Build history of the part. All positions in model axes, mm. Face numbers are marked on the shaded views. Give positions to 0.01 mm unless a question says otherwise; leave off trailing zeros. Order: outer loops, then holes, each group sorted by start corner. A loop starts at its lowest first (then second) coordinate and runs counter-clockwise, first axis right, second up. Notation, with made-up numbers: (44.5, -18.75) - (56.5, -18.75) arc R18 ccw to (56.5, -10.75) - close; hole circle Ø2 at (4.25, 23). An arc over 180 degrees is marked (long way). Answer in a Markdown table with one row per item.
```python
from build123d import *

# Parameters (mm, degrees)
F0_W     = 88.9
F0_H     = 88.9
F0_R     = 1.9812
F0_R_2   = 29.845
F1_DEPTH = 19.05
F2_R     = 3.175
F3_DEPTH = 25.4
F4_R     = 3.175
F5_DEPTH = 25.4


with BuildPart() as f1:
    # F0 (on Top) → F1 (new body)
    with BuildSketch(Plane.XY):
        Rectangle(F0_W, F0_H)
        with Locations((-38.1, -38.1)):
            Circle(F0_R, mode=Mode.SUBTRACT)
        with Locations((38.1, -38.1)):
            Circle(F0_R, mode=Mode.SUBTRACT)
        with Locations((-38.1, 38.1)):
            Circle(F0_R, mode=Mode.SUBTRACT)
        Circle(F0_R_2, mode=Mode.SUBTRACT)
        with Locations((38.1, 38.1)):
            Circle(F0_R, mode=Mode.SUBTRACT)
    extrude(amount=F1_DEPTH)

    # F2 (on face) → F3 (cut)
    with BuildSketch(Plane(origin=(0, 44.45, 0), x_dir=(-1, 0, 0), z_dir=(0, 1, 0))):
        with Locations((0, 9.525)):
            Circle(F2_R)
    extrude(amount=-F3_DEPTH, mode=Mode.SUBTRACT)

    # F4 (on face) → F5 (cut)
    with BuildSketch(Plane(origin=(-44.45, 0, 0), x_dir=(0, -1, 0), z_dir=(-1, 0, 0))):
        with Locations((0, 9.525)):
            Circle(F4_R)
    extrude(amount=-F5_DEPTH, mode=Mode.SUBTRACT)


solid = f1.part
```
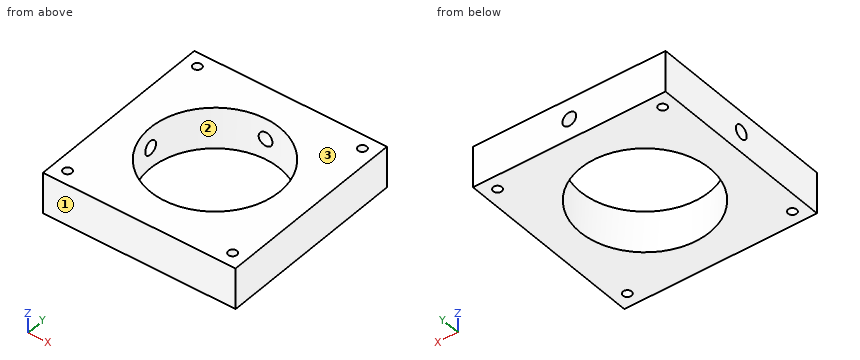
1. Cut at D-D on x = 0. Write the cut outline in (y, z) (3 decimals).
Check result:
| item | result |
|---|---|
| outline | (-44.45, 0) - (-29.845, 0) - (-29.845, 19.05) - (-44.45, 19.05) - close; (29.845, 0) - (44.45, 0) - (44.45, 6.35) - (29.845, 6.35) - close; (29.845, 12.7) - (44.45, 12.7) - (44.45, 19.05) - (29.845, 19.05) - close |
2. Cut at C-C on y = 38.1. Write the cut outline in (x, z) (3 decimals).
Check result:
| item | result |
|---|---|
| outline | (-44.45, 0) - (-40.081, 0) - (-40.081, 19.05) - (-44.45, 19.05) - close; (-36.119, 0) - (36.119, 0) - (36.119, 19.05) - (-36.119, 19.05) - close; (40.081, 0) - (44.45, 0) - (44.45, 19.05) - (40.081, 19.05) - close; hole circle Ø6.35 at (0, 9.525) |
3. Cut at B-B on z = 3. Write the cut outline in (x, y) (3 decimals), and give its area (3 significant figures).
Check result:
| item | result |
|---|---|
| outline | (-44.45, -44.45) - (44.45, -44.45) - (44.45, 44.45) - (-44.45, 44.45) - close; hole circle Ø3.962 at (-38.1, -38.1); hole circle Ø3.962 at (-38.1, 38.1); hole circle Ø59.69 at (0, 0); hole circle Ø3.962 at (38.1, -38.1); hole circle Ø3.962 at (38.1, 38.1) |
| area | 5,060 mm² |
4. Cut at A-A on y = -38.1. Write the cut outline in (x, z).
Check result:
| item | result |
|---|---|
| outline | (-44.45, 0) - (-40.08, 0) - (-40.08, 19.05) - (-44.45, 19.05) - close; (-36.12, 0) - (36.12, 0) - (36.12, 19.05) - (-36.12, 19.05) - close; (40.08, 0) - (44.45, 0) - (44.45, 19.05) - (40.08, 19.05) - close |
5. Drop a flat-ended pin along its axis: P1, Ø5, axis at x = 0, z = 9.525, coming from the +Y side. Give the stop position or say it passes through.
Check result:
| item | result |
|---|---|
| P1 | stops at y = -29.74 |
6. Two-plate mould, pull along Y, no slides. Class the marked faces 1, 2 and 3: +Y half, -Y half, draft (parallel to the pull), parting line (faces both ways), or undercut.
Check result:
| item | result |
|---|---|
| face 1 | -Y half |
| face 2 | undercut |
| face 3 | draft |
7. Probe line 1 (Y direction, x = -38.1, z = 13.25); line 2 (Y direction, x = -39.5, z = 7); line 3 (Y direction, x = 0, z = 4.75) (3 decimals). List the from-to ranges inside material, lowest first.
Check result:
| item | result |
|---|---|
| line 1 | y = -44.45 to -40.08, -36.12 to 36.12, 40.08 to 44.45 |
| line 2 | y = -44.45 to -39.5, -36.7 to -1.92, 1.92 to 36.7, 39.5 to 44.45 |
| line 3 | y = -44.45 to -29.845, 29.845 to 44.45 |
